The listing builds one solid part. Answer for the finished solid, in the listing's coordinates (mm). Face numbers are marked on the shaded views. A direction names the side the tool comes from. Give positions to 0.01 mm unless a question says otherwise; leave off trailing zeros. Loops run counter-clockwise (first coordinate to the right, second up) from the corner with the lowest first, then second, coordinate; pieces in that order, holes last.
Item 1: Section D-D, the plane x = 434.5 is taken. Give the vertices of the cut face in (y, z).
Item 2: Section C-C, the plane z = 11 is taken. Give the vertices of the cut face in (x, y).
Item 3: Section B-B, the plane y = 2 is taken. Give the vertices of the cut face in (x, z), and give its area (3 significant figures).
Item 4: Section A-A, the plane z = 7 is taken. Give the vertices of the cut face in (x, y).
Item 5: Each of these flat-tipped pins is pushed along its axis until it touches: pin 1 Ø12 at (x, y) = (458.5, -17.5) entering from +Z; pin 2 Ø3 at (y, z) = (-8, 8) entering from -X; pin 3 Ø8 at (x, z) = (451, 6) entering from -Y. Where does it stop, or does it pass through?
Item 6: The mould has two halves that part along Y. Classify the marked faces 5, 6, 7 and 8: pulls with the +Y half, pulls with the -Y half, needs draft (parallel to the pull), parting line crosses it, or undercut.
Item 7: A tool of negligible diameter and unlimited length cuts with its end or side. For the marked faces 1, 2, 3 and 4, from which of +Z, -Z, +X, -X, +Y, -Y can it reach the whole face along a straight path? Write none if from no direction.
Item 8: Consider line 1 along Z through (x, y) = (443.5, 0); line 2 along Z through (x, y) = (447.5, 0); line 3 along Z through (x, y) = (446, 5.5). Determine where each line is inside the solid, lowest interval first.
from build123d import *

# Parameters (mm, degrees)
AUFSATZ_LINEAR_START             = -2.5
SKIZZE2_R                        = 25
AUFSATZ_LINEAR_AUSTRAGEN1_DEPTH  = 6
SCHNITT_LINEAR_AUSTRAGEN2_DEPTH  = 476.733381213
AUFSATZ_LINEAR_START_2           = -2.944453
AUFSATZ_LINEAR_AUSTRAGEN5_DEPTH  = 16.944453
SPIEGELN4_START                  = -2.944453335
SPIEGELN4_DEPTH                  = 16.944453335
F_6_4_6_4_DURCHMESSER_BOHRUNG1_D = 6.4


# Read off the part's stored shape, not the designer's step: Spiegeln4
with BuildPart() as part:
    # Skizze2 → Aufsatz-Linear austragen1 (new body)
    with BuildSketch(Plane.XY.offset(AUFSATZ_LINEAR_START)):
        with Locations((450, 0)):
            Circle(SKIZZE2_R)
    extrude(amount=-AUFSATZ_LINEAR_AUSTRAGEN1_DEPTH)

    # Skizze8 → Schnitt-Linear austragen2 (cut, symmetric)
    with BuildSketch(Plane(origin=(0, 0, 0), x_dir=(1, 0, 0), z_dir=(0, 1, 0))):
        with BuildLine():
            Line((450, 2.5), (475, 2.5))
            Line((475, 2.5), (475, 4.284616064))
            ThreePointArc((475, 4.284616064), (462.531808075, 2.946720947), (450, 2.5))
        make_face()
    schnitt_linear_austragen2 = extrude(amount=SCHNITT_LINEAR_AUSTRAGEN2_DEPTH, both=True, mode=Mode.SUBTRACT)

    # Spiegeln1: Schnitt-Linear austragen2 across plane
    add(schnitt_linear_austragen2.mirror(Plane(origin=(450, 0, 0), x_dir=(0, 0, 1), z_dir=(1, 0, 0))), mode=Mode.SUBTRACT)

    # Skizze3 → Aufsatz-Linear austragen5 (add)
    with BuildSketch(Plane.XY.offset(AUFSATZ_LINEAR_START_2)):
        with BuildLine():
            Line((450, 0), (462.5, 0))
            ThreePointArc((462.5, 0), (460.303300859, 5.303300859), (455, 7.5))
            Line((455, 7.5), (450, 7.5))
            Line((450, 7.5), (450, 0))
        make_face()
    extrude(amount=AUFSATZ_LINEAR_AUSTRAGEN5_DEPTH)

    # Spiegeln4 outline → Spiegeln4 (add)
    with BuildSketch(Plane.XY.offset(SPIEGELN4_START)):
        with BuildLine():
            ThreePointArc((455, -7.5), (460.303300859, -5.303300859), (462.5, 0))
            Line((462.5, 0), (450, 0))
            Line((450, 0), (450, 7.5))
            Line((450, 7.5), (445, 7.5))
            ThreePointArc((445, 7.5), (437.5, 0), (445, -7.5))
            Line((445, -7.5), (455, -7.5))
        make_face()
    extrude(amount=SPIEGELN4_DEPTH)

    # Skizze4 → Rotation1 (revolve)
    with BuildSketch(Plane(origin=(450, 0, 0), x_dir=(0, 0, -1), z_dir=(1, 0, 0)), mode=Mode.PRIVATE) as rotation1_sk:
        Polygon((9.5, 7), (8.5, 7), (8.5, 0), (18.5, 0), (18.5, 4), (18.5, 5), (9.5, 5), align=None)
    revolve(rotation1_sk.sketch.rotate(Axis((450, 0, -8.5), (0, 0, -1)), 90), axis=Axis((450, 0, -8.5), (0, 0, -1)))

    # Ø6.4 (6.4) Durchmesser Bohrung1 (through all)
    with Locations(Plane(origin=(462.5, 0, 0), x_dir=(0, 0, -1), z_dir=(1, 0, 0))):
        with Locations((-7, 0)):
            Hole(F_6_4_6_4_DURCHMESSER_BOHRUNG1_D / 2)


solid = part.part
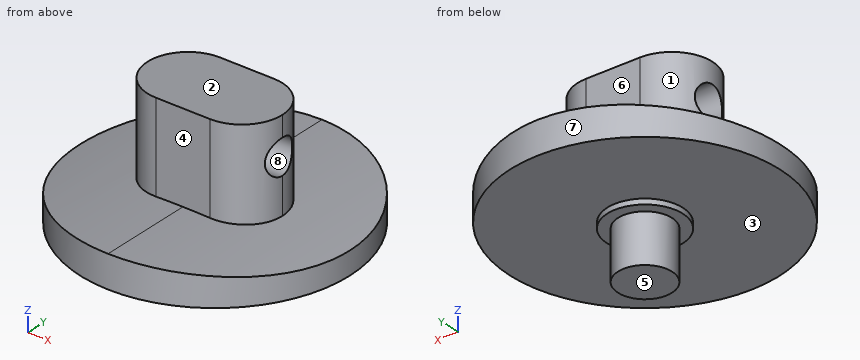
Worked answers:
1. outline: (-19.62, -8.5) - (19.62, -8.5) - (19.62, -3.18) - (-19.62, -3.18) - close
2. outline: (445, -7.5) - (455, -7.5) arc R7.5 ccw to (455, 7.5) - (445, 7.5) arc R7.5 ccw to start
3. outline: (425.08, -8.5) - (443.29, -8.5) - (443.29, -9.5) - (445.42, -9.5) - (445.42, -18.5) - (454.58, -18.5) - (454.58, -9.5) - (456.71, -9.5) - (456.71, -8.5) - (474.92, -8.5) - (474.92, -4.27) arc R176 ccw to (462.23, -2.93) - (462.23, 4.5) - (437.77, 4.5) - (437.77, -2.93) arc R176 ccw to (425.08, -4.27) - close; (437.77, 9.5) - (462.23, 9.5) - (462.23, 14) - (437.77, 14) - close
3. area: 650 mm2
4. outline: (438.22, -3.2) arc R7.5 ccw to (445, -7.5) - (455, -7.5) arc R7.5 ccw to (461.78, -3.2) - close; (438.22, 3.2) - (461.78, 3.2) arc R7.5 ccw to (455, 7.5) - (445, 7.5) arc R7.5 ccw to start
5. pin 1: stops at z = -2.52
5. pin 2: stops at x = 441.26
5. pin 3: stops at y = -7.5
6. face 5: needs draft
6. face 6: pulls with the +Y half
6. face 7: parting line crosses it
6. face 8: undercut
7. face 1: +Z, -X
7. face 2: +Z, +X, -X, +Y, -Y
7. face 3: -Z
7. face 4: +Z, +X, -X, -Y
8. line 1: z = -9.5 to 3.8, 10.2 to 14
8. line 2: z = -18.5 to 3.8, 10.2 to 14
8. line 3: z = -9.5 to 14
